Geometry check sheet. Reference: the model listing, model coordinates, mm. Face numbers are marked on the shaded views. A direction names the side the tool comes from. Give positions to 0.01 mm unless a question says otherwise; leave off trailing zeros. Loops run counter-clockwise (first coordinate to the right, second up) from the corner with the lowest first, then second, coordinate; pieces in that order, holes last. Notation, with made-up numbers: (59, -14) -> (118, -14) arc R15 ccw to (118, -6) -> close; hole circle Ø8 at (61, 57). An arc over 180 degrees is marked (long way). Answer as a JSON object with one key per item and string values.
from build123d import *

# Parameters (mm, degrees)
BOSS_EXTRUDE1_DEPTH                 = 7.5
CBORE_FOR_M3_SHCS1_D                = 3.4
CBORE_FOR_M3_SHCS1_CBORE_D          = 6.5
CBORE_FOR_M3_SHCS1_CBORE_DEPTH      = 3
M6_CLEARANCE_HOLE1_D                = 6.4
TAP_DRILL_FOR_M2X0_4_TAP1_D         = 1.6
TAP_START                           = 6.604
TAP_DRILL_FOR_M4X0_7_TAP1_OUTLINE_R = 1.65
TAP_DRILL_FOR_M4X0_7_TAP1_DEPTH     = 13.396


# Read off the part's stored shape, not the designer's step: Tap Drill for M4x0.7 Tap1
with BuildPart() as part:
    # Sketch1 → Boss-Extrude1 (new, symmetric)
    with BuildSketch(Plane(origin=(0, 0, 0), x_dir=(1, 0, 0), z_dir=(0, 1, 0))):
        Polygon((-6.604, 0), (6.604, 0), (6.604, 20), (20, 20), (20, -7.5), (-20, -7.5), (-20, 20), (-6.604, 20), align=None)
    extrude(amount=BOSS_EXTRUDE1_DEPTH, both=True)

    # CBORE for M3 SHCS1 (through all)
    with Locations(Plane.XY.offset(7.5)):
        with Locations((-12.5, 0), (12.5, 0)):
            CounterBoreHole(CBORE_FOR_M3_SHCS1_D / 2, CBORE_FOR_M3_SHCS1_CBORE_D / 2, CBORE_FOR_M3_SHCS1_CBORE_DEPTH)

    # M6 Clearance Hole1 (through all)
    with Locations(Plane.XY.offset(7.5)):
        with Locations((0, 0)):
            Hole(M6_CLEARANCE_HOLE1_D / 2)

    # Tap Drill for M2x0.4 Tap1 (through all)
    with Locations(Plane(origin=(0, 7.5, 0), x_dir=(1, 0, 0), z_dir=(0, 1, 0))):
        with Locations((0, -3.75)):
            Hole(TAP_DRILL_FOR_M2X0_4_TAP1_D / 2)

    # Tap Drill for M4x0.7 Tap1 outline → Tap Drill for M4x0.7 Tap1 (cut)
    with BuildSketch(Plane.YZ.offset(TAP_START)):
        with Locations((0, -10)):
            Circle(TAP_DRILL_FOR_M4X0_7_TAP1_OUTLINE_R)
    extrude(amount=TAP_DRILL_FOR_M4X0_7_TAP1_DEPTH, mode=Mode.SUBTRACT)


solid = part.part
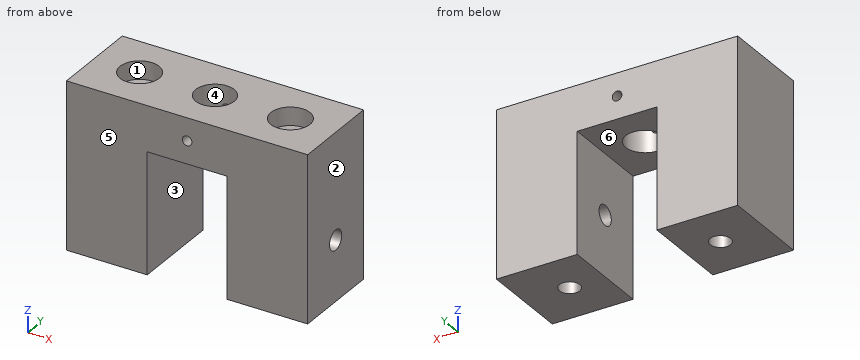
1) Section check C-C on x = -12.5. Record the cut outline in (y, z).
Geometry check:
{"outline": "(-7.5, -20) -> (-1.7, -20) -> (-1.7, 4.5) -> (-3.25, 4.5) -> (-3.25, 7.5) -> (-7.5, 7.5) -> close; (1.7, -20) -> (7.5, -20) -> (7.5, 7.5) -> (3.25, 7.5) -> (3.25, 4.5) -> (1.7, 4.5) -> close"}
2) Depth check by flat-ended pin: P1, Ø4.5, axis at y = 0, z = -10, coming from the +X side; P2, Ø2, axis at x = 12.5, y = 0, coming from the -Z side; P3, Ø2, axis at x = 14, y = 1, coming from the +Z side. Enter the tip coordinate at first touch or a pass-through.
Geometry check:
{"P1": "stops at x = 20", "P2": "passes through", "P3": "stops at z = 4.5"}
3) Material ranges on line 1 along Z through (x, y) = (15, 0); line 2 along X through (y, z) = (6.75, -17.25); line 3 along Y through (x, z) = (8.2, -10), recorded low to high. Write a range as from..to.
Geometry check:
{"line 1": "z = -20..-11.65, -8.35..4.5", "line 2": "x = -20..-6.6, 6.6..20", "line 3": "y = -7.5..-1.65, 1.65..7.5"}
4) Section check B-B on z = -15.25. Record the cut outline in (x, y), plus the area to 3 significant figures.
Geometry check:
{"outline": "(-20, -7.5) -> (-6.6, -7.5) -> (-6.6, 7.5) -> (-20, 7.5) -> close; (6.6, -7.5) -> (20, -7.5) -> (20, 7.5) -> (6.6, 7.5) -> close; hole circle Ø3.4 at (-12.5, 0); hole circle Ø3.4 at (12.5, 0)", "area": "384 mm2"}
5) Section check A-A on z = -10. Record the cut outline in (x, y).
Geometry check:
{"outline": "(-20, -7.5) -> (-6.6, -7.5) -> (-6.6, 7.5) -> (-20, 7.5) -> close; (6.6, -7.5) -> (20, -7.5) -> (20, -1.65) -> (12.91, -1.65) arc R1.7 cw to (12.09, -1.65) -> (6.6, -1.65) -> close; (6.6, 1.65) -> (12.09, 1.65) arc R1.7 cw to (12.91, 1.65) -> (20, 1.65) -> (20, 7.5) -> (6.6, 7.5) -> close; hole circle Ø3.4 at (-12.5, 0)"}
6) Section check D-D on y = -2.5. Record the cut outline in (x, z).
Geometry check:
{"outline": "(-20, -20) -> (-6.6, -20) -> (-6.6, 0) -> (-2, 0) -> (-2, 7.5) -> (-10.42, 7.5) -> (-10.42, 4.5) -> (-14.58, 4.5) -> (-14.58, 7.5) -> (-20, 7.5) -> close; (2, 0) -> (6.6, 0) -> (6.6, -20) -> (20, -20) -> (20, 7.5) -> (14.58, 7.5) -> (14.58, 4.5) -> (10.42, 4.5) -> (10.42, 7.5) -> (2, 7.5) -> close"}
7) Tool access check on the marked faces 1, 2 and 3. Record the directions out of +Z, -Z, +X, -X, +Y, -Y that give a thin tool (end or side, any length) a straight path to the whole face; none if there is none.
Geometry check:
{"face 1": "+Z", "face 2": "+Z, -Z, +X, +Y, -Y", "face 3": "-Z, +Y, -Y"}
8) Draft check along Y on the marked faces 4, 5 and 6. Enter one of: pulls with the +Y half, pulls with the -Y half, needs draft (parallel to the pull), parting line crosses it, or undercut.
Geometry check:
{"face 4": "undercut", "face 5": "pulls with the -Y half", "face 6": "needs draft"}
